Read the model definition and answer for the solid it produces. Units are mm, in the model's axes. A direction names the side the tool comes from. Coordinates: 2 decimals unless noted, no trailing zeros. Write each loop counter-clockwise with the first axis right and the second up, starting at its lowest first coordinate (ties: lowest second). Pieces come first, ordered by that corner, then holes.
1) The part is cut by section A-A (z = 77). Give the number of separate pieces and of enclosed holes in the cut face, then the cut area to 3 significant figures.
2) Determine the mould class of faces 1 (the face through (30.43, 148.55, 196.99)), 2 (the face through (126.75, 2.85, 3.01)), 3 (the face through (120.44, 364.7, 113.95)) for opening direction Z: +Z half, -Z half, draft (parallel to the pull), parting line (faces both ways), or undercut.
3) Each of these flat-tipped pins is pushed along its axis until it touches: pin 1 Ø8 at (y, z) = (5.5, 56) entering from -X; pin 2 Ø1 at (x, y) = (119, 329) entering from +Z; pin 3 Ø6 at (x, z) = (59, 135) entering from +Y. Where does it stop, or does it pass through?
4) Which of the six approach directions +Z, -Z, +X, -X, +Y, -Y give full straight-line access (tool end or side, diameter ignored) to faces 4 (the face through (123, 157, 0)), 5 (the face through (238, 5, 99)), 6 (the face through (126.64, 381.64, 98.74)), 7 (the face through (125, 330, 50))?
5) Find the intervals of material crossed by line 1 (Y direction, x = 107.5, z = 99.5); line 2 (Z direction, x = 111, y = 312); line 3 (Z direction, x = 117, y = 190.5), in increasing order.
6) The part is cut by section B-B (x = 125). Determine the outline of the cut face in (y, z).
from build123d import *

# Parameters (mm, degrees)
BOSS_EXTRUDE1_DEPTH = 200
SKETCH3_R           = 25
CUT_EXTRUDE2_DEPTH  = 150
FILLET1_R           = 10
FILLET2_R           = 10
SHELL1_START        = 10
SHELL1_OUTLINE_R    = 35
SHELL1_DEPTH        = 180
SHELL1_2_OUTLINE_R  = 35
SHELL1_2_DEPTH      = 30
SKETCH4_W           = 226
SKETCH4_H           = 180
CUT_EXTRUDE4_DEPTH  = 10


# Read off the part's stored shape, not the designer's step: Shell1
with BuildPart() as part:
    # Sketch1 → Boss-Extrude1 (new body)
    with BuildSketch(Plane.XY):
        with BuildLine():
            Line((0, 0), (250, 0))
            Line((250, 0), (194.398287, 300))
            ThreePointArc((194.398287, 300), (125, 391.661115), (55.601713, 300))
            Line((55.601713, 300), (0, 0))
        make_face()
    extrude(amount=BOSS_EXTRUDE1_DEPTH)

    # Sketch3 → Cut-Extrude2 (cut)
    with BuildSketch(Plane.XY.offset(200)):
        with Locations((125, 330)):
            Circle(SKETCH3_R)
    extrude(amount=-CUT_EXTRUDE2_DEPTH, mode=Mode.SUBTRACT)

    # Fillet1
    fillet1_edges = [part.edges().sort_by_distance(p)[0] for p in [
        (222.199143, 150, 200),
        (125, 391.661115, 200),
        (100, 330, 200),
        (27.800857, 150, 200),
        (125, 0, 200),
    ]]
    fillet(fillet1_edges, radius=FILLET1_R)

    # Fillet2
    fillet2_edges = [part.edges().sort_by_distance(p)[0] for p in [
        (125, 391.661115, 0),
        (222.199143, 150, 0),
        (125, 0, 0),
        (27.800857, 150, 0),
    ]]
    fillet(fillet2_edges, radius=FILLET2_R)

    # Shell1 outline → Shell1 (cut)
    with BuildSketch(Plane.XY.offset(SHELL1_START)):
        with BuildLine():
            Line((65.875786, 300.559892), (12.023693, 10))
            Line((12.023693, 10), (237.976307, 10))
            Line((237.976307, 10), (184.124214, 300.559892))
            ThreePointArc((184.124214, 300.559892), (125, 381.661115), (65.875786, 300.559892))
        make_face()
        with Locations((125, 330)):
            Circle(SHELL1_OUTLINE_R, mode=Mode.SUBTRACT)
    extrude(amount=SHELL1_DEPTH, mode=Mode.SUBTRACT)

    # Shell1 2 outline → Shell1 2 (cut)
    with BuildSketch(Plane.XY.offset(SHELL1_START)):
        with Locations((125, 330)):
            Circle(SHELL1_2_OUTLINE_R)
    extrude(amount=SHELL1_2_DEPTH, mode=Mode.SUBTRACT)

    # Sketch4 → Cut-Extrude4 (cut)
    with BuildSketch(Plane.XZ):
        with Locations((125, 100)):
            Rectangle(SKETCH4_W, SKETCH4_H)
    extrude(amount=-CUT_EXTRUDE4_DEPTH, mode=Mode.SUBTRACT)


solid = part.part
Reported:
1. separate pieces: 2
1. enclosed holes: 1
1. area: 10,500 mm2
2. face 1: +Z half
2. face 2: -Z half
2. face 3: undercut
3. pin 1: stops at x = 0.28
3. pin 2: stops at z = 50
3. pin 3: stops at y = 354.63
4. face 4: -Z, +X, -X, +Y, -Y
4. face 5: -Y
4. face 6: none
4. face 7: +Z
5. line 1: y = 299.69 to 312.15, 347.85 to 360.31, 379.14 to 389.51
5. line 2: z = 0 to 10, 40 to 50
5. line 3: z = 0 to 10, 190 to 200
6. outline: (0, 10) arc R10 ccw to (10, 0) - (381.66, 0) arc R10 ccw to (391.66, 10) - (391.66, 190) arc R10 ccw to (381.66, 200) - (365, 200) arc R10 ccw to (355, 190) - (355, 50) - (305, 50) - (305, 190) arc R10 ccw to (295, 200) - (10, 200) arc R10 ccw to (0, 190) - (295, 190) - (295, 40) - (365, 40) - (365, 190) - (381.66, 190) - (381.66, 10) - close
